```python
from build123d import *

# Parameters (mm, degrees)
SKETCH1_R           = 55
BOSS_EXTRUDE1_DEPTH = 20
SKETCH2_R           = 45
SKETCH2_R_2         = 30
CUT_EXTRUDE2_DEPTH  = 10
SKETCH4_R           = 15
CUT_EXTRUDE3_DEPTH  = 87
FILLET1_R           = 5
CHAMFER1_SIZE       = 3


with BuildPart() as part:
    # Sketch1 → Boss-Extrude1 (new, symmetric)
    with BuildSketch(Plane.XY):
        Circle(SKETCH1_R)
    extrude(amount=BOSS_EXTRUDE1_DEPTH, both=True)

    # Sketch2 → Cut-Extrude2 (cut)
    with BuildSketch(Plane.XY.offset(20)):
        Circle(SKETCH2_R)
        Circle(SKETCH2_R_2, mode=Mode.SUBTRACT)
    cut_extrude2 = extrude(amount=-CUT_EXTRUDE2_DEPTH, mode=Mode.SUBTRACT)

    # Mirror1: Cut-Extrude2 across plane
    add(cut_extrude2.mirror(Plane.XY), mode=Mode.SUBTRACT)

    # Sketch4 → Cut-Extrude3 (cut)
    with BuildSketch(Plane.XY.offset(20)):
        Circle(SKETCH4_R)
    extrude(amount=-CUT_EXTRUDE3_DEPTH, mode=Mode.SUBTRACT)

    # Fillet1
    fillet1_edges = [part.edges().sort_by_distance(p)[0] for p in [
        (-55, 0, -20),
        (-55, 0, 20),
    ]]
    fillet(fillet1_edges, radius=FILLET1_R)

    # Chamfer1
    chamfer1_edges = [part.edges().sort_by_distance(p)[0] for p in [
        (-30, 0, -20),
        (-45, 0, 10),
        (-30, 0, 10),
        (-30, 0, 20),
    ]]
    chamfer(chamfer1_edges, length=CHAMFER1_SIZE)


solid = part.part
```
Input: part model. Units: mm. Frame: model coordinates. A direction names the side the tool comes from. Round coordinates to 2 decimals unless told otherwise and drop trailing zeros. Loops run counter-clockwise (first coordinate to the right, second up) from the corner with the lowest first, then second, coordinate; pieces in that order, holes last. Notation, with made-up numbers: (43, 79.25) - (55, 79.25) arc R26 cw to (55, 95.25) - close; hole circle Ø7 at (71.5, -14). An arc over 180 degrees is marked (long way). One line per item, written item: value. Start each with the question number.
(1) Section A-A, the plane z = 8. Return loops of the section in (x, y).
(2) Access query for faces 4 (the cylindrical face through (-29.97, 1.32, 15.03)), 5 (the flat face through (-41, 19, 20)), 6 (the flat face through (29, -9, -10)). Directions: +Z, -Z, +X, -X, +Y, -Y. A direction counts if a zero-diameter tool reaches every point of the face in a straight line with its end or side. Return the directions, or none.
(3) Contact query for flat-ended pins moving along their axis: P1, Ø6, axis at x = -36, z = 6.5, coming from the +Y side; P2, Ø4, axis at x = -19.5, z = -2.5, coming from the -Y side; P3, Ø4, axis at y = -34, z = -1.5, coming from the +X side. Output: stop coordinate, or through.
(4) Draft query along Y for faces 1 (the cylindrical face through (20.765, -39.923, -15.07)), 2 (the cylindrical face through (-11.923, -53.692, 0.21)), 3 (the flat face through (12, -12, -20)). Return one class per face: +Y half, -Y half, draft (parallel to the pull), parting line (faces both ways), or undercut.
(5) Ray query, line 1 (Y direction, x = 0, z = -9); line 2 (Y direction, x = -27, z = -13); line 3 (X direction, y = -1.5, z = 13.5) (3 decimals). Return the intervals inside material, ascending. Write a range as [from, to].
Results below:
1. outline: circle Ø110 at (0, 0); hole circle Ø30 at (0, 0)
2. face 4: +Z
2. face 5: +Z, +X, -X, +Y, -Y
2. face 6: -Z
3. P1: y = 44
3. P2: y = -52.14
3. P3: x = 44.73
4. face 1: undercut
4. face 2: parting line
4. face 3: draft
5. line 1: [-55, -15], [15, 55]
5. line 2: [-47.92, -36], [-13.08, 13.08], [36, 47.92]
5. line 3: [-54.98, -44.975], [-29.962, -14.925], [14.925, 29.962], [44.975, 54.98]
